Autodesk Inventor part; units mm, degrees
ref_plane "YZ Plane" through (0, 0, 0) normal (1, 0, 0) x (0, 1, 0)
ref_plane "XZ Plane" through (0, 0, 0) normal (0, 1, 0) x (-1, 0, 0)
ref_plane "XY Plane" through (0, 0, 0) normal (0, 0, 1) x (1, 0, 0)
sketch "Sketch1" plane through (0, 0, 0) normal (0, 1, 0) x (-1, 0, 0)
  line L0 (20, 45) -> (-20, 45)
  line L1 (-20, 45) -> (-20, -45)
  line L2 (-20, -45) -> (20, -45)
  line L3 (20, -45) -> (20, 45)
  line L4 (20, 45) -> (-20, -45) construction
  line L5 (-20, 45) -> (20, -45) construction
  arc A0 (-20, -45) -> (20, -45) centre (0, -45) ccw
  line L6 (20, -45) -> (20, -45)
  line L7 (20, -45) -> (20, 45)
  line L8 (20, 45) -> (20, 45)
  line L9 (20, 45) -> (20, -45)
  line L10 (-20, 45) -> (-50, 45)
  line L11 (-50, 45) -> (-50, -45)
  line L12 (-50, -45) -> (-20, -45)
  line L13 (-20, -45) -> (-20, 45)
  point P0 (0, 0)
  dimension "d0" = 40
  dimension "d1" = 90
  dimension "d7" = 0
  dimension "d8" = 90
  dimension "d35" = 30
extrude "Extrusion1" add sketch "Sketch1" along normal blind 3.6
sketch "Sketch2" plane through (0, 3.6, 0) normal (0, 1, 0) x (1, 0, 0)
  arc A0 (20, 45) -> (-20, 45) centre (0, 45) ccw
  circle A1 centre (0, 45) radius 5.15
  point P0 (0, 0)
  dimension "d4" = 10.3
extrude "Extrusion2" cut sketch "Sketch2" against normal blind 3.6
sketch "Sketch3" plane through (0, 0, 0) normal (0, -1, 0) x (1, 0, 0)
  line L0 (-20, 45) -> (50, 45)
  line L1 (-11.5, 45) -> (18, 45)
  line L2 (18, 45) -> (18, -30)
  line L3 (18, -30) -> (-11.5, -30)
  line L4 (-11.5, -30) -> (-11.5, 45)
  circle A0 centre (28, 20) radius 16.25
  line L5 (-20, -45) -> (-20, 45)
  line L6 (50, 45) -> (50, -45)
  point P0 (0, 0)
  point P1 (16, 45)
  dimension "d10" = 29.5
  dimension "d11" = 75
  dimension "d13" = 32.5
  dimension "d15" = 25
  dimension "d37" = 32
  dimension "d39" = 22
extrude "Extrusion3" cut sketch "Sketch3" against normal blind 10
fillet "Fillet2" radius 2 3 edges at (18, 1.8, 45) (18, 1.8, 32.8087) (18, 1.8, 7.1913)
fillet "Fillet3" radius 4 4 edges at (50, 1.8, 45) (-20, 1.8, 45) (20, 1.8, -45) (-20, 1.8, -45)
chamfer "Chamfer1" distance 20 angle 45 1 edges at (50, 1.8, -45)
fillet "Fillet4" radius 10 2 edges at (30, 1.8, -45) (50, 1.8, -25)
sketch "Sketch6" plane through (3.0674, 0, -14.7029) normal (0, -1, 0) x (1, 0, 0)
  circle A0 centre (21.9326, -26.7971) radius 1.5
  circle A1 centre (43.4326, -6.7971) radius 1.5
  circle A2 centre (43.4326, 56.2029) radius 1.5
  line L0 (25.8579, -30.2971) -> (23.6643, -30.2971)
  line L1 (46.9326, 55.7029) -> (46.9326, -5.2971)
  line L2 (-23.0674, -30.2971) -> (-23.0674, 55.7029)
  line L3 (-16, 59.7029) -> (42.9326, 59.7029)
  circle A3 centre (18.4326, 43) radius 1.75
  line L4 (-23.0674, -30.2971) -> (-23.0674, 55.7029)
  line L5 (16.9326, 59.7029) -> (42.9326, 59.7029)
  line L6 (46.9326, 55.7029) -> (46.9326, -6.155)
  line L7 (22.7905, -30.2971) -> (20.5969, -30.2971)
  point P0 (0, 0)
  dimension "d56" = 3
  dimension "d53" = 3
  dimension "d50" = 3
  dimension "d58" = 3.5
  dimension "d55" = 3.5
  dimension "d57" = 25
  dimension "d54" = 20
  dimension "d52" = 3.5
  dimension "d51" = 3.5
  dimension "d45" = 3.5
  dimension "d46" = 25
  dimension "d62" = 0
  dimension "d63" = 0
  dimension "d64" = 0
  dimension "d65" = 0
  dimension "d66" = 0
  dimension "d67" = 0
  dimension "d68" = 25
  dimension "d69" = 0
  dimension "d70" = 0
extrude "Extrusion6" cut sketch "Sketch6" against normal blind 10
sketch "Sketch7" plane through (33.0492, 0, -22.6689) normal (0, -1, 0) x (1, 0, 0)
  circle A0 centre (-49.5492, 64.1689) radius 1.5
  circle A1 centre (-49.5492, -0.8311) radius 1.5
  line L0 (-49.0492, 67.6689) -> (12.9508, 67.6689)
  line L1 (-53.0492, -23.8754) -> (-53.0492, 41)
  arc A2 (-53.0492, -23.8754) -> (-46.6341, -27.064) centre (-49.0492, -23.8754) ccw
  line L2 (-53.0492, -22.3311) -> (-53.0492, 63.6689)
  line L3 (-49.0492, 67.6689) -> (-44.5492, 67.6689)
  point P0 (0, 0)
  dimension "d74" = 3
  dimension "d71" = 3
  dimension "d76" = 3.5
  dimension "d75" = 3.5
  dimension "d73" = 3.5
  dimension "d72" = 65
  dimension "d80" = 0
  dimension "d81" = 0
extrude "Extrusion7" cut sketch "Sketch7" against normal blind 10
sketch "Sketch8" plane through (0, 0, 0) normal (0, -1, 0) x (1, 0, 0)
  point P0 (0, 0)
sketch "Sketch9" plane through (0, 3.6, 0) normal (0, 1, 0) x (1, 0, 0)
  line L0 (20, -45) -> (46, -45)
  line L1 (50, -41) -> (50, 20.8579)
  line L2 (18, -43) -> (18, -45.6174)
  arc A0 (18, -43) -> (20, -45) centre (20, -43) ccw
  arc A1 (18, -45.6174) -> (39.4564, -45) centre (28, -20) ccw
  arc A2 (50, -36.5) -> (50, -3.5) centre (28, -20) ccw
  point P0 (0, 0)
  dimension "d82" = 25
  dimension "d83" = 22
extrude "Extrusion8" add sketch "Sketch9" against normal blind 3.6
fillet "Fillet5" radius 2 4 edges at (18, 1.8, 45.6174) (50, 1.8, 36.5) (50, 1.8, 3.5) (39.4564, 1.8, 45)
properties part number "p1"
Check sheet for the modelled part. Datum: model origin and axes. Units: mm. A direction names the side the tool comes from. Give positions to 0.01 mm unless a question says otherwise; leave off trailing zeros. Loops run counter-clockwise (first coordinate to the right, second up) from the corner with the lowest first, then second, coordinate; pieces in that order, holes last. Notation, with made-up numbers: M 0.25,-13.5 L 58.25,-13.5 A24 ccw 58.25,4.5 Z; hole C 28.5,8.25 d8. An arc over 180 degrees is marked long. Answer in a Markdown table with one row per item.
1) Cross-section at D-D (z = -37.5). Enter the section's corners in (x, y), plus the area to 3 significant figures.
Solutions:
| item | result |
|---|---|
| outline | M -20,0 L 37.5,0 L 37.5,3.6 L -20,3.6 Z |
| area | 207 mm^2 |
2) Thickness scan on line 1 (Z direction, x = 0, y = 1.5); line 2 (X direction, y = 1.25, z = 20); line 3 (Z direction, x = -16.5, y = 2.25). Record the ranges inside material, lowest first.
Solutions:
| item | result |
|---|---|
| line 1 | z = -65 to -50.15, -39.85 to -30 |
| line 2 | x = -20 to -11.5, 44.25 to 55.5 |
| line 3 | z = -56.3 to -25, -22 to 40, 43 to 44.97 |
3) Depth check by flat-ended pin: pin 1 (1.1 mm diameter, centred on x = 2, y = 2.5, fed in from +Z); pin 2 (5 mm diameter, centred on x = -5.5, z = -53, fed in from -Y); pin 3 (1.8 mm diameter, centred on x = 46.5, z = 41.5, fed in from -Y); pin 4 (1.1 mm diameter, centred on y = 1.5, z = -6, fed in from +X). Enter the tip coordinate at first touch or a pass-through.
Solutions:
| item | result |
|---|---|
| pin 1 | stops at z = -30 |
| pin 2 | stops at y = 0 |
| pin 3 | passes through |
| pin 4 | stops at x = 50 |
4) Cross-section at A-A (z = 20). Enter the section's corners in (x, y), plus the area to 3 significant figures.
Solutions:
| item | result |
|---|---|
| outline | M -20,0 L -11.5,0 L -11.5,3.6 L -20,3.6 Z; M 44.25,0 L 55.5,0 L 55.5,3.6 L 44.25,3.6 Z |
| area | 71.1 mm^2 |
5) Cross-section at C-C (y = 1.65). Count the separate pieces of the cut face and the enclosed holes in it, plus the area to 3 significant figures.
Solutions:
| item | result |
|---|---|
| separate pieces | 1 |
| enclosed holes | 6 |
| area | 3,830 mm^2 |
6) Mould release check, pull along X, two halves, no side actions. Record for faces 4 (the face through (-18.859, 1.825, 43.797)), 5 (the face through (18, 2, 40)), 6 (the face through (40, 2, -35)), 7 (the face through (43, 2, 45)): released by +X, released by -X, zero draft, split by the parting line, or undercut.
Solutions:
| item | result |
|---|---|
| face 4 | released by -X |
| face 5 | undercut |
| face 6 | released by +X |
| face 7 | zero draft |
7) Cross-section at B-B (x = 0). Enter the section's corners in (y, z).
Solutions:
| item | result |
|---|---|
| outline | M 0,-65 L 3.6,-65 L 3.6,-50.15 L 0,-50.15 Z; M 0,-39.85 L 3.6,-39.85 L 3.6,-30 L 0,-30 Z |
8) Tool access check on faces 1 (the face through (-14, 2, 45)), 2 (the face through (-11.5, 2, 7)), 3 (the face through (25, 2, -45)). Record the directions out of +Z, -Z, +X, -X, +Y, -Y that give a thin tool (end or side, any length) a straight path to the whole face; none if there is none.
Solutions:
| item | result |
|---|---|
| face 1 | +Z, -X, +Y, -Y |
| face 2 | +Z, +Y, -Y |
| face 3 | -Z, +X, +Y, -Y |
